Can you work these out from the model? Positions are in its coordinate system, mm. A direction names the side the tool comes from. Give positions to 0.01 mm unless a question says otherwise; leave off trailing zeros. Order: outer loops, then holes, each group sorted by start corner. A loop starts at its lowest first (then second) coordinate and runs counter-clockwise, first axis right, second up. Notation, with made-up numbers: (24.25, -14) -> (36.25, -14) arc R10 cw to (36.25, -6) -> close; hole circle Ø7 at (38.5, 7.5). An arc over 180 degrees is marked (long way). Answer as CSV lines item,"result".
```python
from build123d import *

# Parameters (mm, degrees)
SKETCH1_W               = 100
SKETCH1_H               = 75
BOSS_EXTRUDE1_DEPTH     = 60
CUT_EXTRUDE1_DEPTH      = 87.638617256
CUT_EXTRUDE1_DEPTH_BACK = 40
CUT_EXTRUDE2_DEPTH      = 87.638617256
CUT_EXTRUDE2_DEPTH_BACK = 20


with BuildPart() as part:
    # Sketch1 → Boss-Extrude1 (new body)
    with BuildSketch(Plane(origin=(0, 0, 0), x_dir=(1, 0, 0), z_dir=(0, 1, 0))):
        Rectangle(SKETCH1_W, SKETCH1_H)
    extrude(amount=BOSS_EXTRUDE1_DEPTH)

    # Sketch2 → Cut-Extrude1 (cut, two sides: drawn at the far end of the back side and taken through both)
    with BuildSketch(Plane(origin=(0, 60, 0), x_dir=(1, 0, 0), z_dir=(0, 1, 0)).offset(-CUT_EXTRUDE1_DEPTH_BACK)):
        Polygon((-25, -259.632034356), (-25, -37.5), (-25, -12.5), (25, -12.5), (25, 37.5), (25, 259.632034356), (467.218719806, 217.050740324), (417.218719806, -302.213328388), align=None)
    extrude(amount=CUT_EXTRUDE1_DEPTH + CUT_EXTRUDE1_DEPTH_BACK, mode=Mode.SUBTRACT)

    # Sketch3 → Cut-Extrude2 (cut, two sides: drawn at the far end of the back side and taken through both)
    with BuildSketch(Plane(origin=(0, 60, 0), x_dir=(1, 0, 0), z_dir=(0, 1, 0)).offset(-CUT_EXTRUDE2_DEPTH_BACK)):
        Polygon((-25, -234.632034356), (-25, -12.5), (-25, 12.5), (25, 12.5), (25, 37.5), (25, 259.632034356), (467.008191751, 214.918264963), (417.008191751, -279.345803749), align=None)
    extrude(amount=CUT_EXTRUDE2_DEPTH + CUT_EXTRUDE2_DEPTH_BACK, mode=Mode.SUBTRACT)


solid = part.part
```
Item 1: Imagine slicing it at C-C, the plane x = -23.5. Please give me the cut outline in (y, z), then the cut area to 3 significant figures.
Numbers:
outline,"(0, -37.5) -> (60, -37.5) -> (60, -12.5) -> (40, -12.5) -> (40, 12.5) -> (20, 12.5) -> (20, 37.5) -> (0, 37.5) -> close"
area,"3,000 mm²"
Item 2: Imagine slicing it at D-D, the plane z = -22.5. Please give me the cut outline in (x, y), then the cut area to 3 significant figures.
Numbers:
outline,"(-50, 0) -> (50, 0) -> (50, 20) -> (25, 20) -> (25, 60) -> (-50, 60) -> close"
area,"5,000 mm²"
Item 3: Please list where these lines run through material, in increasing order: line 1 along Y through (x, z) = (-10.5, 24); line 2 along Z through (x, y) = (-20.5, 53); line 3 along X through (y, z) = (28, 16).
Numbers:
line 1,"y = 0 to 20"
line 2,"z = -37.5 to -12.5"
line 3,"x = -50 to -25"
Item 4: For faces 1 (the flat face through (-12, 30, -37.5)), 2 (the flat face through (25, 35, -18)), 3 (the flat face through (0, 30, 12.5)), which set-ups out of +Z, -Z, +X, -X, +Y, -Y let a thin tool reach every point of the face, with its end or its side?
Numbers:
face 1,"-Z, +X, -X, +Y, -Y"
face 2,"+Z, -Z, +X, +Y"
face 3,"+Z, +X, +Y"
Item 5: Imagine slicing it at B-B, the plane y = 23.5. Please give me the cut outline in (x, z).
Numbers:
outline,"(-50, -37.5) -> (25, -37.5) -> (25, 12.5) -> (-25, 12.5) -> (-25, 37.5) -> (-50, 37.5) -> close"
Item 6: Imagine slicing it at A-A, the plane z = 2.5. Please give me the cut outline in (x, y), then the cut area to 3 significant figures.
Numbers:
outline,"(-50, 0) -> (50, 0) -> (50, 20) -> (25, 20) -> (25, 40) -> (-25, 40) -> (-25, 60) -> (-50, 60) -> close"
area,"4,000 mm²"
Item 7: For pin 1 (4 mm diameter, centred on x = 24, z = 14, fed in from +Y); pin 2 (10 mm diameter, centred on x = -2, y = 32.5, fed in from +Z); pin 3 (6 mm diameter, centred on x = -10, y = 49, fed in from +Z), each with a flat end and sliding along its axis, tell me the tip position at first contact or that it passes through.
Numbers:
pin 1,"stops at y = 40"
pin 2,"stops at z = 12.5"
pin 3,"stops at z = -12.5"
